```python
from build123d import *

# Parameters (mm, degrees)
F0_R     = 15
F1_DEPTH = 3
F2_R     = 10.9
F2_R_2   = 5
F3_DEPTH = 5.8
F4_DEPTH = 25
F5_DEPTH = 40.4
F6_SIZE  = 1


with BuildPart() as f1:
    # F0 (on Top) → F1 (new body)
    with BuildSketch(Plane.XY):
        Circle(F0_R)
    extrude(amount=F1_DEPTH)

    # F2 (on Top) → F3 (join)
    with BuildSketch(Plane.XY):
        Circle(F2_R)
        Circle(F2_R_2, mode=Mode.SUBTRACT)
    extrude(amount=F3_DEPTH)

    # F4 (add): a face of the model
    f4_faces = [f1.faces().sort_by_distance(p)[0] for p in [
        (0, 0, 3),
    ]]
    extrude(f4_faces, amount=F4_DEPTH)

    # F5 (cut): a face of the model
    f5_faces = [f1.faces().sort_by_distance(p)[0] for p in [
        (0, 0, 28),
    ]]
    extrude(f5_faces, amount=-F5_DEPTH, mode=Mode.SUBTRACT)

    # F6
    f6_edges = [f1.edges().sort_by_distance(p)[0] for p in [
        (-15, 0, 0),
        (-10.9, 0, 5.8),
    ]]
    chamfer(f6_edges, length=F6_SIZE)


solid = f1.part
```
Verification items for the finished model (mm, model axes). A direction names the side the tool comes from. Give positions to 0.01 mm unless a question says otherwise; leave off trailing zeros. Order: outer loops, then holes, each group sorted by start corner. A loop starts at its lowest first (then second) coordinate and runs counter-clockwise, first axis right, second up. Notation, with made-up numbers: (15.5, 11) -> (41.5, 11) arc R34 cw to (41.5, 48) -> close; hole circle Ø4 at (53.5, -28.75). An arc over 180 degrees is marked (long way). Use a Markdown table: item, result.
1) Section check A-A, the plane x = 0. Record the boundary of the cut face in (y, z).
Results:
| item | result |
|---|---|
| outline | (-15, 1) -> (-14, 0) -> (-5, 0) -> (-5, 5.8) -> (-9.9, 5.8) -> (-10.9, 4.8) -> (-10.9, 3) -> (-15, 3) -> close; (5, 0) -> (14, 0) -> (15, 1) -> (15, 3) -> (10.9, 3) -> (10.9, 4.8) -> (9.9, 5.8) -> (5, 5.8) -> close |
2) Section check C-C, the plane z = 2.05. Record the boundary of the cut face in (x, y), then the cut area to 3 significant figures.
Results:
| item | result |
|---|---|
| outline | circle Ø30 at (0, 0); hole circle Ø10 at (0, 0) |
| area | 628 mm² |
3) Material ranges on probe 1 along Y at (x, z) = (0, 4.45); probe 2 along Z at (x, y) = (10.5, -8.5); probe 3 along X at (y, z) = (2.75, 5.5), recorded low to high.
Results:
| item | result |
|---|---|
| probe 1 | -10.9 to -5, 5 to 10.9 |
| probe 2 | 0 to 3 |
| probe 3 | -9.82 to -4.18, 4.18 to 9.82 |
4) Mould release check, pull along Y, two halves, no side actions. Record for faces 3 (the cylindrical face through (-1.08, 4.88, 2.94)), 4 (the cylindrical face through (-14.985, 0.66, 1.986)), 5 (the flat face through (10, 5, 3)): pulls with the +Y half, pulls with the -Y half, needs draft (parallel to the pull), parting line crosses it, or undercut.
Results:
| item | result |
|---|---|
| face 3 | undercut |
| face 4 | parting line crosses it |
| face 5 | needs draft |
5) Depth check by flat-ended pin: pin 1 Ø9 at (x, y) = (0.5, 2.5) entering from +Z; pin 2 Ø6 at (x, y) = (0, 0) entering from -Z; pin 3 Ø2 at (x, z) = (5.5, 5) entering from +Y; pin 4 Ø8 at (x, y) = (-9.5, -11) entering from +Z. Enter the tip coordinate at first touch or a pass-through.
Results:
| item | result |
|---|---|
| pin 1 | z = 5.8 |
| pin 2 | through |
| pin 3 | y = 9.92 |
| pin 4 | z = 5.17 |
6) Tool access check on faces 1 (the flat face through (0, -6, 0)), 2 (the cylindrical face through (10.4, 3.27, 3.89)). Record the directions out of +Z, -Z, +X, -X, +Y, -Y that give a thin tool (end or side, any length) a straight path to the whole face; none if there is none.
Results:
| item | result |
|---|---|
| face 1 | -Z, +X, -X, +Y, -Y |
| face 2 | +Z |
